```python
from build123d import *


with BuildPart() as part:
    # Sketch → Revolution (revolve)
    with BuildSketch(Plane.XZ):
        with BuildLine():
            Line((-16.25, 33), (-16.25, 3))
            Line((-16.25, 3), (-3.5, 3))
            ThreePointArc((-3, 2.5), (-3.146447, 2.853553), (-3.5, 3))
            Line((-3, 2.5), (-3, 1))
            ThreePointArc((-4, 0), (-3.292893, 0.292893), (-3, 1))
            Line((-4, 0), (-16.25, 0))
            Line((-19.25, 3), (-16.25, 0))
            Line((-19.25, 3), (-19.25, 31.5))
            Line((-17.45, 33.3), (-19.25, 31.5))
            Line((-17.45, 33.3), (-16.55, 33.3))
            Line((-16.25, 33), (-16.55, 33.3))
        make_face()
    revolve(axis=Axis((0, 0, 0), (0, 0, 1)))


solid = part.part
```
Check sheet for the modelled part. Datum: model origin and axes. Units: mm. Round coordinates to 2 decimals unless told otherwise and drop trailing zeros. Loops run counter-clockwise (first coordinate to the right, second up) from the corner with the lowest first, then second, coordinate; pieces in that order, holes last. Notation, with made-up numbers: (67, 13) - (114, 13) arc R36 ccw to (114, 49) - close; hole circle Ø11 at (28.25, -33.5). An arc over 180 degrees is marked (long way). Write item = value, one per line. Start each with the question number.
Q1. Release check for a two-part mould opening along Y. For faces 1 (the face through (0, -4, 3)), 2 (the face through (13.011, 9.977, 0.146)), 3 (the face through (-15.5, -4.88, 17.79)), 4 (the face through (3, 3, 0)) record: pulls with the +Y half, pulls with the -Y half, needs draft (parallel to the pull), parting line crosses it, or undercut.
Q2. Section check C-C (z = 16). Record the boundary of the cut face in (x, y).
Q3. Thickness scan on L1, parallel to X at y = 0, z = 9; L2, parallel to Y at x = 11.5, z = 18.5. Record the ranges inside material, lowest first.
Q4. Section check A-A (y = 0). Record the boundary of the cut face in (x, z), plus the area to 3 significant figures.
Q5. Depth check by flat-ended pin: P1, Ø1, axis at y = -13, z = 22.5, coming from the +X side; P2, Ø1.5, axis at x = -2.5, z = 15.5, coming from the +Y side; P3, Ø12, axis at x = 5.5, y = -8, coming from the +Z side; P4, Ø10, axis at y = 2, z = 17, coming from the -X side. Enter the tip coordinate at first touch or a pass-through.
Derived:
q1.face_1 = undercut
q1.face_2 = parting line crosses it
q1.face_3 = undercut
q1.face_4 = needs draft
q2.outline = circle Ø38.5 at (0, 0); hole circle Ø32.5 at (0, 0)
q3.L1 = -19.25 to -16.25, 16.25 to 19.25
q3.L2 = -15.44 to -11.48, 11.48 to 15.44
q4.outline = (-19.25, 3) - (-16.25, 0) - (-4, 0) arc R1 ccw to (-3, 1) - (-3, 2.5) arc R0.5 ccw to (-3.5, 3) - (-16.25, 3) - (-16.25, 33) - (-16.55, 33.3) - (-17.45, 33.3) - (-19.25, 31.5) - close; (3, 1) arc R1 ccw to (4, 0) - (16.25, 0) - (19.25, 3) - (19.25, 31.5) - (17.45, 33.3) - (16.55, 33.3) - (16.25, 33) - (16.25, 3) - (3.5, 3) arc R0.5 ccw to (3, 2.5) - close
q4.area = 266 mm^2
q5.P1 = 14.64
q5.P2 = 19.17
q5.P3 = 3
q5.P4 = -19.25
